Job drawing, mm, ordinate dimensions from the low corner. One solid piece. A direction names the side the tool comes from. Give positions to 0.01 mm unless a question says otherwise; leave off trailing zeros. Order: outer loops, then holes, each group sorted by start corner. A loop starts at its lowest first (then second) coordinate and runs counter-clockwise, first axis right, second up. Notation, with made-up numbers: M 52.5,82.5 L 88.5,82.5 A26 cw 88.5,116.5 Z; hole C -21,28.25 d9. An arc over 180 degrees is marked long. Use CSV: the item, a comma, the result in double quotes. Start each with the question number.
Item 1: Band-saw the part on D-D on y = 3.25. Give the number of separate pieces and of enclosed holes in the cut face, plus the area to 3 significant figures.
Item 2: Two-plate mould, pull along X, no slides. Class the marked faces 3 and 4: pulls with the +X half, pulls with the -X half, needs draft (parallel to the pull), parting line crosses it, or undercut.
Item 3: Band-saw the part on B-B on x = 147.5. Write the cut outline in (y, z), plus the area to 3 significant figures.
Item 4: Band-saw the part on A-A on z = 71.5. Write the cut outline in (x, y).
Item 5: Which spindle directions (+Z, -Z, +X, -X, +Y, -Y) get a long thin tool onto all of the face, cutting with end or side? Do the marked faces 1 and 2. Say none if no direction does.
Item 6: Band-saw the part on C-C on z = 12.5. Write the cut outline in (x, y).
Item 7: Wall check: line 1 along X through (y, z) = (3.5, 91.5); line 2 along Z through (x, y) = (147.5, 5.5); line 3 along X through (y, z) = (6.5, 71.5). Give the ranges that are in metal, low to high.
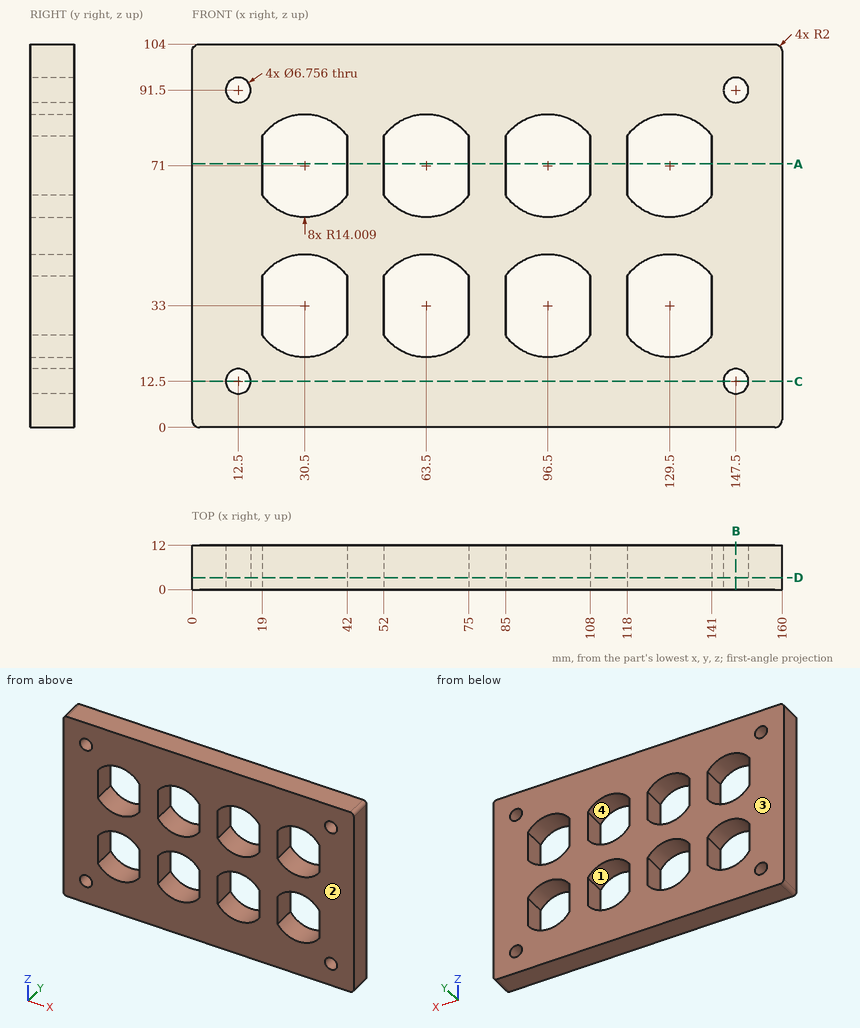
Model answer:
1,separate pieces,"1"
1,enclosed holes,"12"
1,area,"12,000 mm^2"
2,face 3,"needs draft"
2,face 4,"undercut"
3,outline,"M 0,0 L 12,0 L 12,9.12 L 0,9.12 Z; M 0,15.88 L 12,15.88 L 12,88.12 L 0,88.12 Z; M 0,94.88 L 12,94.88 L 12,104 L 0,104 Z"
3,area,"1,090 mm^2"
4,outline,"M 0,0 L 19,0 L 19,12 L 0,12 Z; M 42,0 L 52,0 L 52,12 L 42,12 Z; M 75,0 L 85,0 L 85,12 L 75,12 Z; M 108,0 L 118,0 L 118,12 L 108,12 Z; M 141,0 L 160,0 L 160,12 L 141,12 Z"
5,face 1,"+Y, -Y"
5,face 2,"+Z, -Z, +X, -X, -Y"
6,outline,"M 0,0 L 9.12,0 L 9.12,12 L 0,12 Z; M 15.88,0 L 144.12,0 L 144.12,12 L 15.88,12 Z; M 150.88,0 L 160,0 L 160,12 L 150.88,12 Z"
7,line 1,"x = 0 to 9.12, 15.88 to 144.12, 150.88 to 160"
7,line 2,"z = 0 to 9.12, 15.88 to 88.12, 94.88 to 104"
7,line 3,"x = 0 to 19, 42 to 52, 75 to 85, 108 to 118, 141 to 160"
